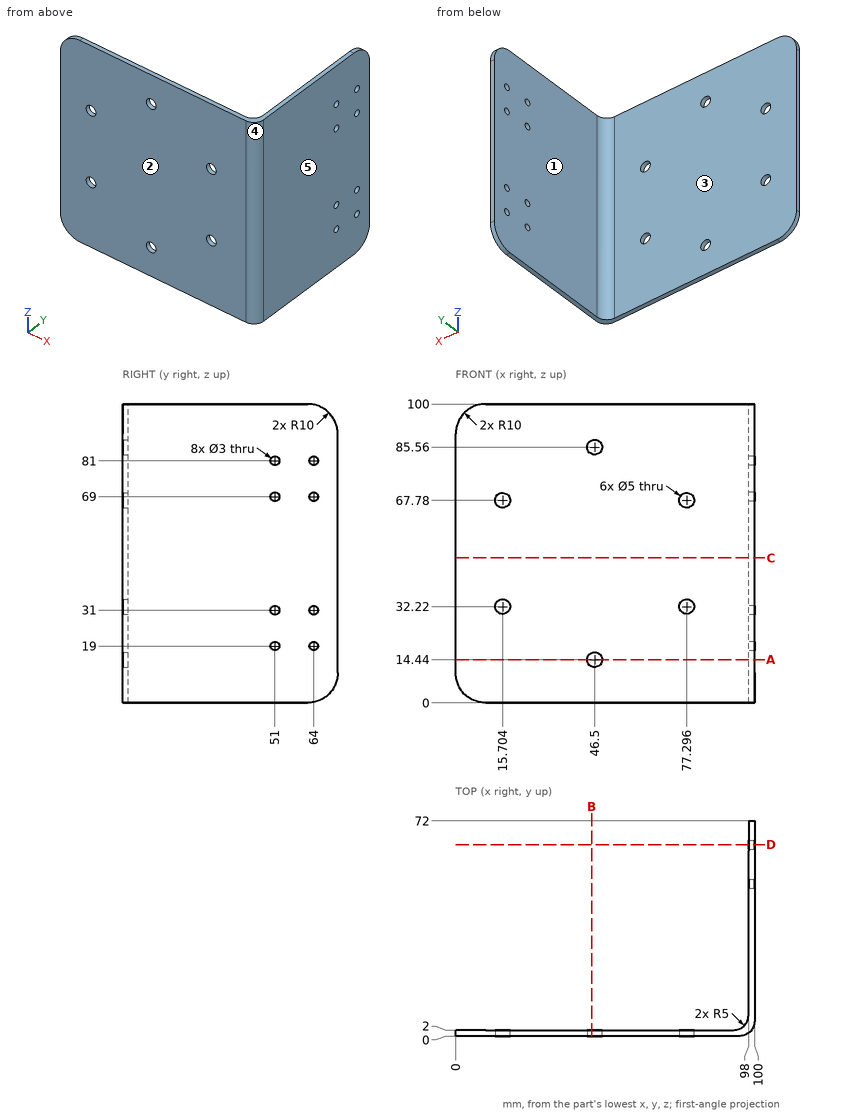
Part print with two shaded views. Sizes in mm from the minimum x, y, z corner. A direction names the side the tool comes from. Round coordinates to 2 decimals unless told otherwise and drop trailing zeros. Order: outer loops, then holes, each group sorted by start corner. A loop starts at its lowest first (then second) coordinate and runs counter-clockwise, first axis right, second up. Notation, with made-up numbers: M 40,-15 L 56,-15 A26 ccw 56,3 Z; hole C 36,20.25 d5. An arc over 180 degrees is marked long. Put each result on its own line as item: value. Start each with the question number.
1. Two-plate mould, pull along Y, no slides. Class the marked faces 3, 4 and 5: +Y half, -Y half, draft (parallel to the pull), parting line (faces both ways), or undercut.
2. Slice it at D-D on y = 64. List the corners of the cut face in (x, z), then the cut area to 3 significant figures.
3. Slice it at A-A on z = 14.44. List the corners of the cut face in (x, y), then the cut area to 3 significant figures.
4. Slice it at C-C on z = 48.5. List the corners of the cut face in (x, y), then the cut area to 3 significant figures.
5. Tool access for the marked faces 1 and 2: list every direction of +Z, -Z, +X, -X, +Y, -Y with a clear straight run to the whole face (end or side of a thin tool).
6. Drill centre lines: probe 1 along Z at (x, y) = (99, 51); probe 2 along Y at (x, z) = (99, 69); probe 3 along Z at (x, y) = (46.5, 1). Where is each one in solid material? Low to high. Write a range as [from, to].
7. Slice it at B-B on x = 45.5. List the corners of the cut face in (y, z).
8. Drop flat-ended pins along their axis: pin 1 (2.5 mm diameter, centred on y = 51, z = 31, fed in from +X); pin 2 (4 mm diameter, centred on x = 89.5, z = 74, fed in from +Y); pin 3 (4 mm diameter, centred on y = 25.5, z = 76.5, fed in from -X); pin 4 (4 mm diameter, centred on y = 64, z = 31, fed in from +X). Give the stop position or say it passes through.
Findings:
1. face 3: +Y half
1. face 4: -Y half
1. face 5: draft
2. outline: M 98,0.2 L 100,0.2 L 100,17.5 L 98,17.5 Z; M 98,20.5 L 100,20.5 L 100,29.5 L 98,29.5 Z; M 98,32.5 L 100,32.5 L 100,67.5 L 98,67.5 Z; M 98,70.5 L 100,70.5 L 100,79.5 L 98,79.5 Z; M 98,82.5 L 100,82.5 L 100,99.8 L 98,99.8 Z
2. area: 175 mm2
3. outline: M 0,0 L 44,0 L 44,2 L 0,2 Z; M 49,0 L 95,0 A5 ccw 100,5 L 100,72 L 98,72 L 98,7 A5 cw 93,2 L 49,2 Z
3. area: 330 mm2
4. outline: M 0,0 L 95,0 A5 ccw 100,5 L 100,72 L 98,72 L 98,7 A5 cw 93,2 L 0,2 Z
4. area: 340 mm2
5. face 1: +Z, -Z, -X, +Y
5. face 2: +Z, -Z, +X, -X, -Y
6. probe 1: [0, 17.5], [20.5, 29.5], [32.5, 67.5], [70.5, 79.5], [82.5, 100]
6. probe 2: [2, 49.5], [52.5, 62.5], [65.5, 72]
6. probe 3: [0, 11.94], [16.94, 83.06], [88.06, 100]
7. outline: M 0,0 L 2,0 L 2,12.15 L 0,12.15 Z; M 0,16.73 L 2,16.73 L 2,83.27 L 0,83.27 Z; M 0,87.85 L 2,87.85 L 2,100 L 0,100 Z
8. pin 1: through
8. pin 2: y = 2
8. pin 3: x = 98
8. pin 4: x = 100
